from build123d import *

# Parameters (mm, degrees)
SKETCH_2_R               = 4
EXTRUDE_1_DEPTH          = 10
CHAMFER_1_SIZE           = 3.5
CUT_EXTRUDE_1_DEPTH      = 12.489125293
CUT_EXTRUDE_1_DEPTH_BACK = 12.489125293
SKETCH_4_W               = 4
SKETCH_4_H               = 1.2


# Read off the part's stored shape, not the designer's step: M8 机械螺纹 螺柱1
with BuildPart() as part:
    # 草图2 → 凸台-拉伸1 (new body)
    with BuildSketch(Plane.XY):
        Circle(SKETCH_2_R)
    extrude(amount=EXTRUDE_1_DEPTH)

    # M8 机械螺纹 螺柱1 outline → M8 机械螺纹 螺柱1 (revolve, cut)
    with BuildSketch(Plane.XZ):
        Polygon((4, 10), (3.3235, 10), (4, 9.3235), align=None)
    revolve(axis=Axis((0, 0, 0), (0, 0, 1)), mode=Mode.SUBTRACT)

    # 倒角1
    chamfer_1_edges = [part.edges().sort_by_distance(p)[0] for p in [
        (-4, 0, 0),
    ]]
    chamfer(chamfer_1_edges, length=CHAMFER_1_SIZE)

    # 草图4 → 切除-拉伸1 (cut, two sides: drawn at the far end of the back side and taken through both)
    with BuildSketch(Plane(origin=(0, 0, 0), x_dir=(0, 0, -1), z_dir=(1, 0, 0)).offset(-CUT_EXTRUDE_1_DEPTH_BACK)):
        with Locations((-10, 0)):
            Rectangle(SKETCH_4_W, SKETCH_4_H)
    extrude(amount=CUT_EXTRUDE_1_DEPTH + CUT_EXTRUDE_1_DEPTH_BACK, mode=Mode.SUBTRACT)


solid = part.part
Check sheet for the modelled part. Datum: model origin and axes. Units: mm. A direction names the side the tool comes from. Coordinates: 2 decimals unless noted, no trailing zeros. Loops run counter-clockwise (first coordinate to the right, second up) from the corner with the lowest first, then second, coordinate; pieces in that order, holes last. Notation, with made-up numbers: (46.25, 32) -> (82.25, 32) arc R28 ccw to (82.25, 66) -> close; hole circle Ø7 at (83, -30.75). An arc over 180 degrees is marked (long way). Answer in a Markdown table with one row per item.
1. Access from +Z, -Z, +X, -X, +Y, -Y to the whole of each face (thin tool, end or side, straight path). Record for faces 1 (the face through (3.695, -1.532, 6.371)), 2 (the face through (0, 0.6, 9)).
Check values:
| item | result |
|---|---|
| face 1 | +Z, -Z |
| face 2 | +Z, +X, -X |
2. Go/stop test with flat-tipped pins: pin 1 (1.6 mm diameter, centred on x = -0.5, z = 9, fed in from +Y); pin 2 (3 mm diameter, centred on x = -2.5, z = 6.5, fed in from -Y); pin 3 (1.5 mm diameter, centred on x = 0, y = -1.5, fed in from -Z). Record where each tip stops, or that it passes through.
Check values:
| item | result |
|---|---|
| pin 1 | stops at y = 4 |
| pin 2 | stops at y = -3.87 |
| pin 3 | stops at z = 0.25 |
3. Release check for a two-part mould opening along Y. For faces 3 (the face through (0.07, 3.44, 9.88)), 4 (the face through (0, -0.6, 9)), 5 (the face through (1.01, 0.32, 0.56)) record: released by +Y, released by -Y, zero draft, split by the parting line, or undercut.
Check values:
| item | result |
|---|---|
| face 3 | released by +Y |
| face 4 | undercut |
| face 5 | split by the parting line |
4. Material ranges on line 1 along Z through (x, y) = (0.25, 0); line 2 along Y through (x, z) = (-2.75, 9.75); line 3 along X through (y, z) = (-3, 8), recorded low to high. Write a range as [from, to].
Check values:
| item | result |
|---|---|
| line 1 | z = [0, 8] |
| line 2 | y = [-2.28, -0.6], [0.6, 2.28] |
| line 3 | x = [-2.65, 2.65] |
5. Sectioned sample at B-B, the plane x = 0. Record the boundary of the cut face in (y, z).
Check values:
| item | result |
|---|---|
| outline | (-4, 3.5) -> (-0.5, 0) -> (0.5, 0) -> (4, 3.5) -> (4, 9.32) -> (3.32, 10) -> (0.6, 10) -> (0.6, 8) -> (-0.6, 8) -> (-0.6, 10) -> (-3.32, 10) -> (-4, 9.32) -> close |
6. Sectioned sample at A-A, the plane y = 0. Record the boundary of the cut face in (x, z), then the cut area to 4 significant figures.
Check values:
| item | result |
|---|---|
| outline | (-4, 3.5) -> (-0.5, 0) -> (0.5, 0) -> (4, 3.5) -> (4, 8) -> (-4, 8) -> close |
| area | 51.75 mm2 |
7. Sectioned sample at C-C, the plane z = 9. Record the boundary of the cut face in (x, y).
Check values:
| item | result |
|---|---|
| outline | (-3.95, -0.6) arc R4 ccw to (3.95, -0.6) -> close; (-3.95, 0.6) -> (3.95, 0.6) arc R4 ccw to start |
8. Sectioned sample at D-D, the plane z = 1. Record the boundary of the cut face in (x, y), then the cut area to 3 significant figures.
Check values:
| item | result |
|---|---|
| outline | circle Ø3 at (0, 0) |
| area | 7.07 mm2 |
